Verification items for the finished model (mm, model axes). A direction names the side the tool comes from. Give positions to 0.01 mm unless a question says otherwise; leave off trailing zeros. Loops run counter-clockwise (first coordinate to the right, second up) from the corner with the lowest first, then second, coordinate; pieces in that order, holes last. Notation, with made-up numbers: (75.5, 81.5) - (104.5, 81.5) arc R33 cw to (104.5, 110.5) - close; hole circle Ø11 at (43, 28.5). An arc over 180 degrees is marked (long way). One line per question, with ' | ' between items. Start each with the question number.
1. Depth check by flat-ended pin: pin 1 Ø3 at (y, z) = (3.5, 35.5) entering from +X; pin 2 Ø4 at (x, z) = (-8.5, 108) entering from -Y; pin 3 Ø5 at (y, z) = (-9, 25) entering from +X. Enter the tip coordinate at first touch or a pass-through.
2. Thickness scan on line 1 along X through (y, z) = (-0.5, -11); line 2 along X through (y, z) = (-4, 25); line 3 along Y through (x, z) = (-12, 96). Record the ranges inside material, lowest first. Write a range as from..to.
3. Section check D-D, the plane z = 123.5. Enter the section's corners in (x, y), then the cut area to 3 significant figures.
4. Tool access check on faces 1 (the face through (0, 8.23, 122)), 2 (the face through (5.38, -8.43, 121.37)), 3 (the face through (-5.38, -8.43, -21.37)). Record the directions out of +Z, -Z, +X, -X, +Y, -Y that give a thin tool (end or side, any length) a straight path to the whole face; none if there is none.
5. Mould release check, pull along Z, two halves, no side actions. Record for faces 4 (the face through (-3.7, 16.664, 49.3)), 5 (the face through (0, 0, 136.08)), 6 (the face through (0, 8.23, -21)): +Z half, -Z half, draft (parallel to the pull), parting line (faces both ways), or undercut.
6. Section check C-C, the plane z = 15.5. Enter the section's corners in (x, y), then the cut area to 3 significant figures.
Autodesk Inventor part; units mm, degrees
ref_plane "Plano de trabajo1" through (0, 10, 100) normal (0, 1, 0) x (-1, 0, 0)
ref_plane "YZ Plane" through (0, 0, 0) normal (1, 0, 0) x (0, 1, 0)
ref_plane "XY Plane" through (0, 0, 0) normal (0, 0, 1) x (1, 0, 0)
sketch "Boceto1" plane through (0, 0, 0) normal (0, 0, 1) x (1, 0, 0)
  circle A0 centre (0, 0) radius 17.07
  dimension "d0" = 34.14
extrude "Extrusión1" add sketch "Boceto1" along normal blind 100
sketch "Boceto2" plane through (0, 0, 100) normal (0, 0, 1) x (1, 0, 0)
  circle A0 centre (0, 0) radius 10
  dimension "d3" = 20
extrude "Extrusión2" add sketch "Boceto2" along normal blind 36.08
sketch "Boceto3" plane through (0, 0, 0) normal (0, 0, -1) x (-1, 0, 0)
  circle A0 centre (0, 0) radius 10
  dimension "d6" = 20
extrude "Extrusión3" add sketch "Boceto3" along normal blind 36.08
fillet "Empalme1" radius 7.07 1 edges at (-10, 0, 100)
fillet "Empalme2" radius 7.07 1 edges at (10, 0, 0)
ref_plane "Plano de trabajo1" through (0, 10, 100) normal (0, 1, 0) x (-1, 0, 0)
sketch "Boceto4" plane through (0, 10, 100) normal (0, 1, 0) x (-1, 0, 0)
  line L0 (10, 36.08) -> (-10, 36.08)
  line L1 (-3.5, 34.6498) -> (3.5, 34.6498)
  line L2 (3.5, 34.6498) -> (3.5, 8.6498)
  line L3 (3.5, 8.6498) -> (-3.5, 8.6498)
  line L4 (-3.5, 8.6498) -> (-3.5, 34.6498)
  line L5 (-3.5, 34.6498) -> (3.5, 8.6498) construction
  line L6 (3.5, 34.6498) -> (-3.5, 8.6498) construction
  line L7 (10, -107.07) -> (-10, -107.07)
  line L8 (-10, -136.08) -> (10, -136.08)
  line L9 (10, -107.07) -> (10, -136.08)
  line L10 (-3.5, -108.575) -> (3.5, -108.575)
  line L11 (3.5, -108.575) -> (3.5, -134.575)
  line L12 (3.5, -134.575) -> (-3.5, -134.575)
  line L13 (-3.5, -134.575) -> (-3.5, -108.575)
  point P0 (0, -100)
  point P1 (0, 21.6498)
  dimension "d11" = 7
  dimension "d12" = 26
  dimension "d13" = 7
  dimension "d14" = 26
extrude "Extrusión4" cut sketch "Boceto4" against normal blind 1.77
properties part number "Eje cuñero"
Results list:
1) pin 1: x = 16.95 | pin 2: y = -7.6 | pin 3: x = 15.78
2) line 1: -9.99..9.99 | line 2: -16.59..16.59 | line 3: -12.14..12.14
3) outline: (-3.5, 8.23) - (-3.5, 9.37) arc R10 ccw (long way) to (3.5, 9.37) - (3.5, 8.23) - close | area: 303 mm²
4) face 1: +Y | face 2: +Z | face 3: -Z
5) face 4: draft | face 5: +Z half | face 6: undercut
6) outline: circle Ø34.14 at (0, 0) | area: 915 mm²
